Geometry check sheet. Reference: drawing and pictorial views, mm from the part's lowest x, y, z. Round coordinates to 2 decimals unless told otherwise and drop trailing zeros. Write each loop counter-clockwise with the first axis right and the second up, starting at its lowest first coordinate (ties: lowest second). Pieces come first, ordered by that corner, then holes. Notation, with made-up numbers: M 37,-26.75 L 79,-26.75 A15 cw 79,-5.75 Z; hole C 44.5,85.25 d8. An arc over 180 degrees is marked long. Answer in a Markdown table with one row per item. Add a question column.
1. Sectioned sample at B-B on z = 5.75. Record the cut outline in (x, y), plus the area to 3 significant figures.
2. Sectioned sample at C-C on y = 0.5. Record the cut outline in (x, z), plus the area to 3 significant figures.
3. Material ranges on probe 1 along Y at (x, z) = (13.5, 7); probe 2 along Y at (x, z) = (7.5, 5), recorded low to high.
4. Sectioned sample at A-A on x = 1.75. Record the cut outline in (y, z), plus the area to 3 significant figures.
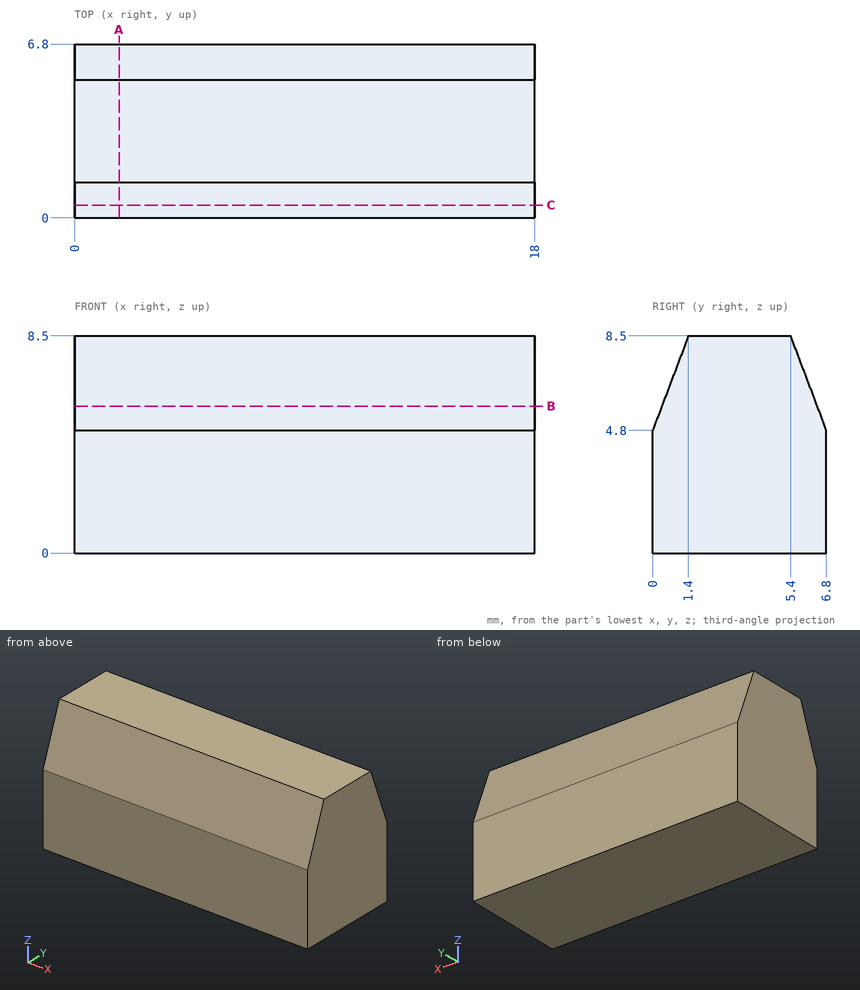
Geometry check:
| question | item | result |
|---|---|---|
| 1 | outline | M 0,0.36 L 18,0.36 L 18,6.44 L 0,6.44 Z |
| 1 | area | 109 mm2 |
| 2 | outline | M 0,0 L 18,0 L 18,6.12 L 0,6.12 Z |
| 2 | area | 110 mm2 |
| 3 | probe 1 | y = 0.83 to 5.97 |
| 3 | probe 2 | y = 0.08 to 6.72 |
| 4 | outline | M 0,0 L 6.8,0 L 6.8,4.8 L 5.4,8.5 L 1.4,8.5 L 0,4.8 Z |
| 4 | area | 52.6 mm2 |
